from build123d import *

# Parameters (mm, degrees)
CUT_EXTRUDE1_DEPTH      = 22.997045256
CUT_EXTRUDE1_DEPTH_BACK = 22.997045256
SKETCH2_R               = 6.35
FILLET1_R               = 1.524
CHAMFER1_SIZE           = 0.381


with BuildPart() as part:
    # Sketch1 → Revolve1 (revolve)
    with BuildSketch(Plane.XY, mode=Mode.PRIVATE) as revolve1_sk:
        with BuildLine():
            Line((-12.7, 0), (12.7, 0))
            Line((12.7, 0), (12.7, 9.525))
            Line((12.7, 9.525), (8.400260413, 9.525))
            ThreePointArc((8.400260413, 9.525), (0, 12.7), (-8.400260413, 9.525))
            Line((-8.400260413, 9.525), (-12.7, 9.525))
            Line((-12.7, 9.525), (-12.7, 0))
        make_face()
    revolve(revolve1_sk.sketch.rotate(Axis((-19.734173111, 0, 0), (1, 0, 0)), 90), axis=Axis((-19.734173111, 0, 0), (1, 0, 0)))

    # Sketch2 → Cut-Extrude1 (cut, two sides: drawn at the far end of the back side and taken through both)
    with BuildSketch(Plane(origin=(0, 0, 0), x_dir=(0, 0, -1), z_dir=(1, 0, 0)).offset(-CUT_EXTRUDE1_DEPTH_BACK)):
        Circle(SKETCH2_R)
    extrude(amount=CUT_EXTRUDE1_DEPTH + CUT_EXTRUDE1_DEPTH_BACK, mode=Mode.SUBTRACT)

    # Fillet1
    fillet1_edges = [part.edges().sort_by_distance(p)[0] for p in [
        (8.400260413, 0, -9.525),
        (-8.400260413, 0, -9.525),
    ]]
    fillet(fillet1_edges, radius=FILLET1_R)

    # Chamfer1
    chamfer1_edges = [part.edges().sort_by_distance(p)[0] for p in [
        (-12.7, 0, 6.35),
        (12.7, 0, 6.35),
        (-12.7, 0, -9.525),
        (12.7, 0, -9.525),
    ]]
    chamfer(chamfer1_edges, length=CHAMFER1_SIZE)


solid = part.part
Design review of the part built by this model. Coordinates are the model's own, in mm. A direction names the side the tool comes from. Coordinates: 2 decimals unless noted, no trailing zeros. Loops run counter-clockwise (first coordinate to the right, second up) from the corner with the lowest first, then second, coordinate; pieces in that order, holes last. Notation, with made-up numbers: M 13.5,87.5 L 35.5,87.5 A13 cw 35.5,102.5 Z; hole C 79,63 d7. An arc over 180 degrees is marked long. Use one line per item in the form item = value.
(1) Clearance check with flat-ended pins moving along their axes: P1, Ø1, axis at x = -8.5, z = -7.5, coming from the -Y side; P2, Ø6, axis at x = 7, y = -1, coming from the +Z side; P3, Ø8, axis at x = -9, y = -7, coming from the +Z side. State where each tip first meets the part, or that it passes through.
Return value:
P1 = -6.65
P2 = 12.03
P3 = 10.32
(2) Consider section B-B (z = -11). Write out the cut boundary in (x, y).
Return value:
outline = C 0,0 d12.69
(3) Draft analysis for pull direction Z (two halves, no side actions). For faces 3 (the face through (10.615, -2.861, 9.085)), 4 (the face through (-0.17, -6.2, 1.38)), 5 (the face through (-12.7, 7, -1)), state which applies: pulls with the +Z half, pulls with the -Z half, needs draft (parallel to the pull), parting line crosses it, or undercut.
Return value:
face_3 = parting line crosses it
face_4 = undercut
face_5 = needs draft
(4) Consider section C-C (x = -3). Write out the cut boundary in (y, z), and give its area (3 significant figures).
Return value:
outline = C 0,0 d24.68; hole C 0,0 d12.7
area = 352 mm2
(5) For faces 1 (the face through (-10.66, 3.65, 8.8)), 2 (the face through (12.7, 7, 1)), list the 3-axis set-ups (+Z, -Z, +X, -X, +Y, -Y) from which the entire face can be reached by the end or side of a thin tool; tool diameter is ignored.
Return value:
face_1 = -X
face_2 = +Z, -Z, +X, +Y, -Y
(6) For line 1 along Y through (x, z) = (3.75, 0); line 2 along Z through (x, y) = (0.5, -1.25); line 3 along Z through (x, y) = (-9.75, -5.5), list the stretches that pass through material, from the lowest coordinate up. Write a range as from..to.
Return value:
line_1 = -12.13..-6.35, 6.35..12.13
line_2 = -12.63..-6.23, 6.23..12.63
line_3 = -7.78..-3.17, 3.17..7.78
(7) Consider section A-A (x = 4.25). Write out the cut boundary in (y, z).
Return value:
outline = C 0,0 d23.94; hole C 0,0 d12.7
